Model file for the job. Use its own axes, mm. Face numbers are marked on the shaded views. Coordinates: 2 decimals unless noted, no trailing zeros. Order: outer loops, then holes, each group sorted by start corner. A loop starts at its lowest first (then second) coordinate and runs counter-clockwise, first axis right, second up. Notation, with made-up numbers: M 0.5,77.25 L 57.5,77.25 A7 ccw 57.5,90.25 Z; hole C -13.75,-14 d6. An arc over 180 degrees is marked long. Return JSON: item names as keys, results as strings.
```python
from build123d import *

# Parameters (mm, degrees)
F1_DEPTH = 609.6
F3_R     = 2.54
F4_R     = 4.7625
F5_DEPTH = 25.4


with BuildPart() as f1:
    # F0 (on Front) → F1 (new body)
    with BuildSketch(Plane.XZ):
        with BuildLine():
            Line((-20.234578, 19.260229), (-1.413178, 19.260229))
            Line((-1.413178, 19.260229), (-1.413178, 20.758829))
            Line((-1.413178, 20.758829), (-20.463178, 20.758829))
            ThreePointArc((-20.463178, 20.758829), (-23.157255, 19.642906), (-24.273178, 16.948829))
            Line((-24.273178, 16.948829), (-24.273178, -23.307944))
            ThreePointArc((-24.273178, -23.307944), (-21.449279, -26.988121), (-17.163621, -25.212944))
            Line((-17.163621, -25.212944), (-10.813621, -14.214421))
            Line((-10.813621, -14.214421), (-12.111447, -13.465121))
            Line((-12.111447, -13.465121), (-18.034874, -23.724797))
            ThreePointArc((-18.034874, -23.724797), (-20.891979, -24.908249), (-22.774578, -22.454797))
            Line((-22.774578, -22.454797), (-22.774578, 16.720229))
            ThreePointArc((-22.774578, 16.720229), (-22.030629, 18.51628), (-20.234578, 19.260229))
        make_face()
    extrude(amount=-F1_DEPTH)

    # F3
    f3_edges = [f1.edges().sort_by_distance(p)[0] for p in [
        (-1.413178, 0, 20.009529),
        (-11.462534, 0, -13.839771),
        (-11.462534, 609.6, -13.839771),
        (-1.413178, 609.6, 20.009529),
    ]]
    fillet(f3_edges, radius=F3_R)

    # F4 (on face) → F5 (cut)
    with BuildSketch(Plane.YZ.offset(-22.774578)):
        with Locations((32.974709, 0)):
            Circle(F4_R)
        with Locations((310.342709, 0)):
            Circle(F4_R)
        with Locations((587.710709, 0)):
            Circle(F4_R)
    extrude(amount=-F5_DEPTH, mode=Mode.SUBTRACT)


solid = f1.part
```
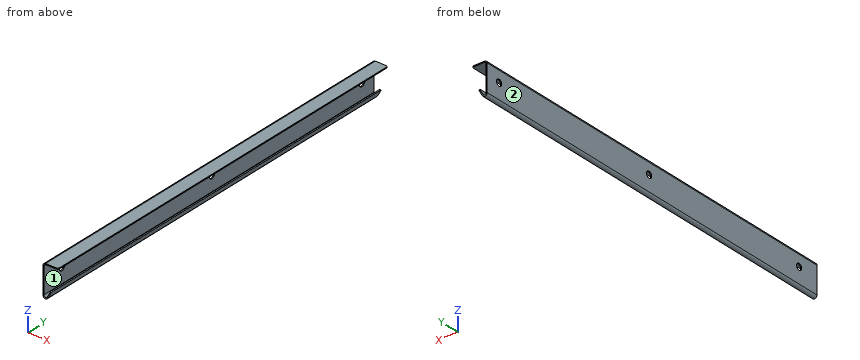
Item 1: Saw through at A-A (y = 341). Write the cut outline in (x, z).
Check result:
{"outline": "M -24.27,-23.31 A3.81 ccw -17.16,-25.21 L -10.81,-14.21 L -12.11,-13.47 L -18.03,-23.72 A2.54 cw -22.77,-22.45 L -22.77,16.72 A2.54 cw -20.23,19.26 L -1.41,19.26 L -1.41,20.76 L -20.46,20.76 A3.81 ccw -24.27,16.95 Z"}
Item 2: Pull direction Z, two halves, no side cores. Call the marked faces 1 and 2: +Z half, -Z half, draft (parallel to the pull), parting line (faces both ways), or undercut.
Check result:
{"face 1": "undercut", "face 2": "draft"}
Item 3: Wall check: line 1 (Z direction, x = -20.25, y = 472); line 2 (X direction, y = 99, z = -21); line 3 (X direction, y = 86, z = -17). Give the ranges that are in metal, low to high.
Check result:
{"line 1": "z = -27.11 to -24.99, 19.26 to 20.76", "line 2": "x = -24.27 to -22.77, -16.46 to -14.73", "line 3": "x = -24.27 to -22.77, -14.15 to -12.42"}
Item 4: Drop flat-ended pins along their axis: pin 1 Ø10 at (x, z) = (-7, -11.5) entering from -Y; pin 2 Ø19.5 at (y, z) = (394, -1) entering from +X; pin 3 Ø1.5 at (x, z) = (-11.5, -17.5) entering from -Y. Give the stop position or say it passes through.
Check result:
{"pin 1": "stops at y = 1.26", "pin 2": "stops at x = -22.77", "pin 3": "passes through"}
